For this review, use the dimensioned drawing (mm, ordinates from the lowest corner) and the shaded views. A direction names the side the tool comes from. Give positions to 0.01 mm unless a question says otherwise; leave off trailing zeros. Write each loop counter-clockwise with the first axis right and the second up, starting at its lowest first coordinate (ties: lowest second). Pieces come first, ordered by that corner, then holes. Notation, with made-up numbers: (21.5, 15.5) - (40.5, 15.5) arc R17 ccw to (40.5, 25.5) - close; hole circle Ø3 at (23, 62.25). An arc over 180 degrees is marked (long way). One line per question, with ' | ' between items. Start each with the question number.
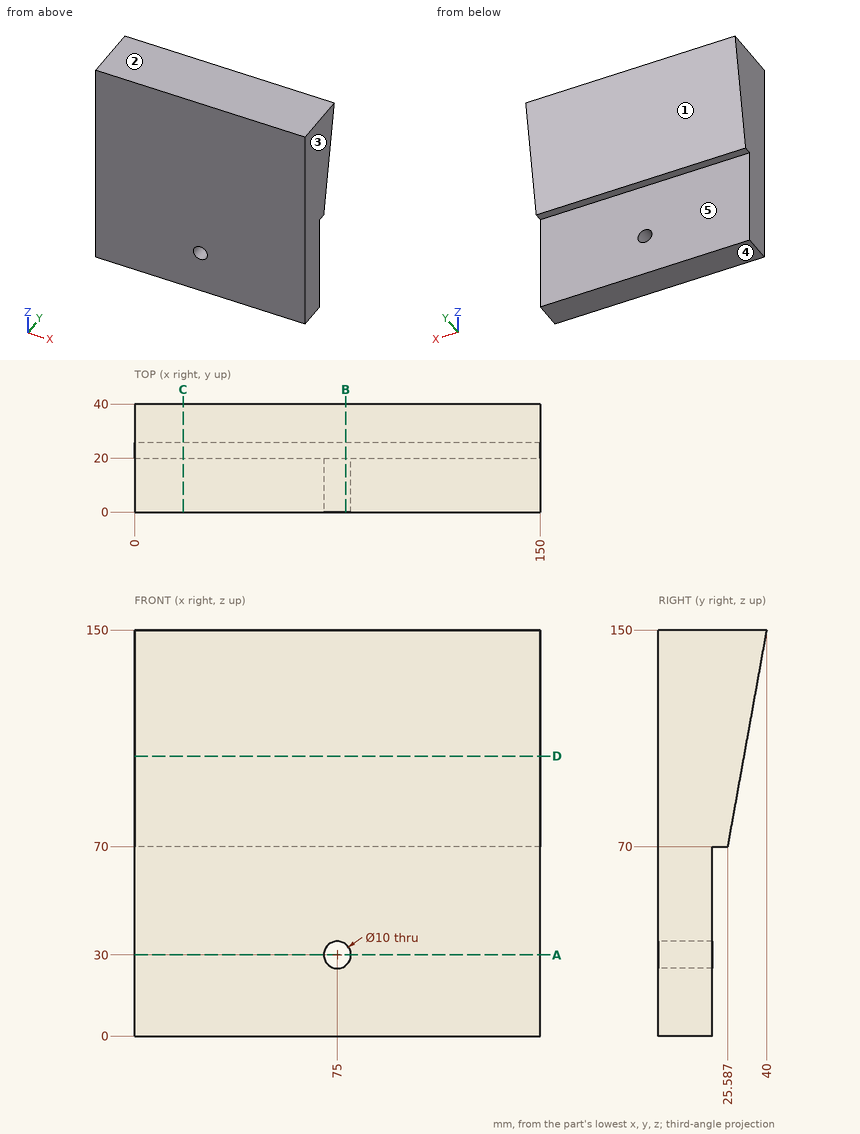
Item 1: For probe 1 along Z at (x, y) = (75, 6.25); probe 2 along Y at (x, z) = (141, 57.5); probe 3 along Z at (x, y) = (23.5, 21), list the stretches that pass through material, from the lowest coordinate up.
Item 2: Take a section at C-C (x = 18). Give the boundary of the cut face in (y, z).
Item 3: Take a section at A-A (z = 30). Give the boundary of the cut face in (x, y).
Item 4: Take a section at B-B (x = 78). Give the boundary of the cut face in (y, z), plus the area to 3 significant figures.
Item 5: Take a section at D-D (z = 103.5). Give the boundary of the cut face in (x, y).
Item 6: Clearance check with flat-ended pins moving along their axes: P1, Ø6, axis at x = 102.5, z = 120, coming from the +Y side; P2, Ø9, axis at x = 75, z = 30, coming from the -Y side; P3, Ø4.5, axis at x = 95, y = 24, coming from the -Z side. State where each tip first meets the part, or that it passes through.
Item 7: Machinability: for the marked faces 4 and 5, which of the approach directions +Z, -Z, +X, -X, +Y, -Y give a long, thin tool a straight path to every point of the face, cutting with its end or side? Answer none if there is none.
Item 8: The part is to be moulded in two halves that separate along Z. For the marked faces 1, 2 and 3, say which applies: +Z half, -Z half, draft (parallel to the pull), parting line (faces both ways), or undercut.
Check sheet entries:
1) probe 1: z = 0 to 25, 35 to 150 | probe 2: y = 0 to 20 | probe 3: z = 70 to 150
2) outline: (0, 0) - (20, 0) - (20, 70) - (25.59, 70) - (40, 150) - (0, 150) - close
3) outline: (0, 0) - (70, 0) - (70, 20) - (0, 20) - close; (80, 0) - (150, 0) - (150, 20) - (80, 20) - close
4) outline: (0, 0) - (20, 0) - (20, 26) - (0, 26) - close; (0, 34) - (20, 34) - (20, 70) - (25.59, 70) - (40, 150) - (0, 150) - close | area: 3,860 mm^2
5) outline: (0, 0) - (150, 0) - (150, 31.62) - (0, 31.62) - close
6) P1: stops at y = 35.14 | P2: passes through | P3: stops at z = 70
7) face 4: -Z, +X, -X, +Y, -Y | face 5: -Z, +X, -X, +Y
8) face 1: -Z half | face 2: +Z half | face 3: draft
